CAD build for the part. Positions are in the model's coordinates, mm. A direction names the side the tool comes from. Round coordinates to 2 decimals unless told otherwise and drop trailing zeros. Loops run counter-clockwise (first coordinate to the right, second up) from the corner with the lowest first, then second, coordinate; pieces in that order, holes last.
from build123d import *

# Parameters (mm, degrees)
F0_R     = 2.5
F0_R_2   = 1.5
F0_R_3   = 11
F2_DEPTH = 8


with BuildPart() as f2:
    # F0 (on Front) → F2 (new body)
    with BuildSketch(Plane.XZ):
        with BuildLine():
            Line((15.7396886074, 65), (0, 65))
            Line((0, 65), (-15.7396886074, 65))
            ThreePointArc((-15.7396886074, 65), (-22.5341845457, 62.3372218819), (-25.7102334624, 55.7669649888))
            Line((-25.7102334624, 55.7669649888), (-30, 0))
            Line((-30, 0), (-16.6938662384, -62.0952908873))
            ThreePointArc((-16.6938662384, -62.0952908873), (-13.202617548, -67.7766608796), (-6.9158420977, -70))
            Line((-6.9158420977, -70), (0, -70))
            Line((0, -70), (6.9158420977, -70))
            ThreePointArc((6.9158420977, -70), (13.202617548, -67.7766608796), (16.6938662384, -62.0952908873))
            Line((16.6938662384, -62.0952908873), (30, 0))
            Line((30, 0), (25.7102334624, 55.7669649888))
            ThreePointArc((25.7102334624, 55.7669649888), (22.5341845457, 62.3372218819), (15.7396886074, 65))
        make_face()
        with BuildLine():
            Line((-2.5, -62), (-2.5, -50))
            ThreePointArc((-2.5, -50), (0, -47.5), (2.5, -50))
            Line((2.5, -50), (2.5, -62))
            ThreePointArc((2.5, -62), (0, -64.5), (-2.5, -62))
        make_face(mode=Mode.SUBTRACT)
        with Locations((-22.5, 9)):
            Circle(F0_R, mode=Mode.SUBTRACT)
        with Locations((-15.5, 26.5)):
            Circle(F0_R_2, mode=Mode.SUBTRACT)
        with Locations((-15.5, 57.5)):
            Circle(F0_R_2, mode=Mode.SUBTRACT)
        with Locations((22.5, 9)):
            Circle(F0_R, mode=Mode.SUBTRACT)
        with Locations((15.5, 26.5)):
            Circle(F0_R_2, mode=Mode.SUBTRACT)
        with Locations((0, 42)):
            Circle(F0_R_3, mode=Mode.SUBTRACT)
        with Locations((15.5, 57.5)):
            Circle(F0_R_2, mode=Mode.SUBTRACT)
    extrude(amount=F2_DEPTH)


solid = f2.part
Item 1: Mould opens along X. For faces 1 (the flat face through (0, -4, -70)), 2 (the flat face through (23.254, -3.944, -31.482)), 3 (the cylindrical face through (-16.61, -3.94, 27.51)) say: released by +X, released by -X, zero draft, split by the parting line, or undercut.
Verdict:
face 1: zero draft
face 2: released by +X
face 3: undercut
Item 2: Cut at A-A (x = 0). List the corners of the cut face in (y, z).
Verdict:
outline: (-8, -70) - (0, -70) - (0, -64.5) - (-8, -64.5) - close; (-8, -47.5) - (0, -47.5) - (0, 31) - (-8, 31) - close; (-8, 53) - (0, 53) - (0, 65) - (-8, 65) - close
Item 3: Cut at D-D (x = 22.5). List the corners of the cut face in (y, z).
Verdict:
outline: (-8, -35) - (0, -35) - (0, 6.5) - (-8, 6.5) - close; (-8, 11.5) - (0, 11.5) - (0, 62.37) - (-8, 62.37) - close
Item 4: Flat gauge pins, fed straight in: P1, Ø4, axis at y = -6, z = -55, coming from the -X side; P2, Ø4, axis at y = -6.5, z = -43.5, coming from the -X side; P3, Ø4, axis at y = -2.5, z = -11, coming from the +X side. Where does each tip first touch, or does it go through?
Verdict:
P1: stops at x = -18.64
P2: stops at x = -21.11
P3: stops at x = 28.07
Item 5: 3-axis set-ups, long thin cutter, end or side, ignore diameter. For faces 4 (the flat face through (0, -4, 65)), 5 (the flat face through (2.5, -4, -56)): which of +Z, -Z, +X, -X, +Y, -Y reach the whole face in a straight line?
Verdict:
face 4: +Z, +X, -X, +Y, -Y
face 5: +Y, -Y
Item 6: Cut at B-B (z = -56). List the corners of the cut face in (x, y), plus the area to 3 significant figures.
Verdict:
outline: (-18, -8) - (-2.5, -8) - (-2.5, 0) - (-18, 0) - close; (2.5, -8) - (18, -8) - (18, 0) - (2.5, 0) - close
area: 248 mm2
Item 7: Wall check: L1, parallel to X at y = -2, z = 26; L2, parallel to Z at x = -10, y = -2.5; L3, parallel to Z at x = -15.5, y = -4.25. Give the ranges that are in metal, low to high.
Verdict:
L1: x = -28 to -16.91, -14.09 to 14.09, 16.91 to 28
L2: z = -69.51 to 37.42, 46.58 to 65
L3: z = -65.13 to 25, 28 to 56, 59 to 65
Item 8: Cut at C-C (y = -1.5). State how many separate pieces and enclosed holes the cut face has, plus the area to 3 significant figures.
Verdict:
separate pieces: 1
enclosed holes: 8
area: 6,140 mm2
